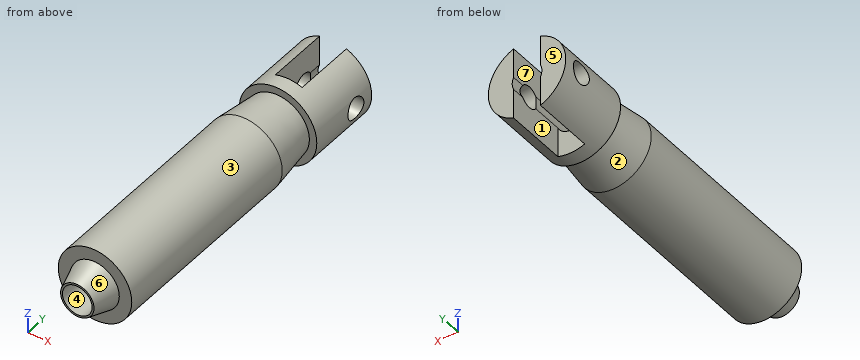
Autodesk Inventor part; units mm, degrees
ref_plane "YZ Plane" through (0, 0, 0) normal (1, 0, 0) x (0, 1, 0)
ref_plane "XZ Plane" through (0, 0, 0) normal (0, 1, 0) x (-1, 0, 0)
ref_plane "XY Plane" through (0, 0, 0) normal (0, 0, 1) x (1, 0, 0)
sketch "Sketch1" plane through (0, 0, 0) normal (0, 0, 1) x (1, 0, 0)
  line L0 (2, 45.442) -> (2, -1.498)
  line L1 (2.254, -1.498) -> (3.2702, 1.754)
  line L2 (3.2702, 1.754) -> (4.953, 1.754)
  line L3 (4.953, 1.754) -> (4.953, 29.3765)
  line L4 (4.953, 29.3765) -> (4.2142, 35.3709)
  line L5 (4.2142, 35.3709) -> (5.2137, 35.3709)
  line L6 (5.2137, 35.3709) -> (5.2137, 45.442)
  line L7 (5.2137, 45.442) -> (2, 45.442)
  line L8 (0, 63.454) -> (0, -29.2362) construction
  line L9 (2.7221, 0) -> (1.4605, -4.0372) construction
  line L10 (1.4605, -4.0372) -> (0, -4.0372) construction
  line L11 (2.254, -1.498) -> (2, -1.498)
  point P0 (0, 0)
  dimension "d0" = 2
  dimension "d1" = 4.953
  dimension "d2" = 3.2702
  dimension "d3" = 43.688
  dimension "d4" = 10.0711
  dimension "d5" = 5.9944
  dimension "d16" = 1.4605
  dimension "d17" = 5.7912
  dimension "d18" = 0.254
revolve "Revolution1" add sketch "Sketch1" angle 360 about axis through (0, 63.454, 0) along (0, -1, 0)
sketch "Sketch2" plane through (0, 45.442, 0) normal (0, 1, 0) x (1, 0, 0)
  line L0 (-1.8097, 6.35) -> (1.8097, 6.35)
  line L1 (1.8097, 6.35) -> (1.8097, -6.35)
  line L2 (1.8097, -6.35) -> (-1.8097, -6.35)
  line L3 (-1.8097, -6.35) -> (-1.8097, 6.35)
  point P0 (0, 0)
  point P1 (0, -6.35)
  point P2 (1.8097, 0)
  dimension "d8" = 3.6195
  dimension "d9" = 12.7
extrude "Extrusion1" cut sketch "Sketch2" against normal blind 8.128
sketch "Sketch3" plane through (1.8097, 45.442, 0.8514) normal (-1, 0, 0) x (0, 0, 1)
  circle A0 centre (-0.8514, -2.8829) radius 1.4605
  line L0 (0, 0) -> (4.0382, 0)
  point P0 (-0.8514, -45.442)
  dimension "d12" = 2.921
  dimension "d13" = 2.8829
extrude "Extrusion2" cut sketch "Sketch3" along normal through all both and the other way through all
properties part number "SolenoidShaft"
For this review, take the finished solid that the model builds, in its own axes (mm). Face numbers are marked on the shaded views. A direction names the side the tool comes from. Round coordinates to 2 decimals unless told otherwise and drop trailing zeros. Order: outer loops, then holes, each group sorted by start corner. A loop starts at its lowest first (then second) coordinate and runs counter-clockwise, first axis right, second up. Notation, with made-up numbers: (9.5, 68) -> (55.5, 68) arc R13 cw to (55.5, 93) -> close; hole circle Ø3 at (42.5, 75). An arc over 180 degrees is marked (long way). Use a Markdown table: item, result.
Item 1: Take a section at D-D (y = 30). State the section outline as (x, z) points, plus the area to 3 significant figures.
Resolved:
| item | result |
|---|---|
| outline | circle Ø9.75 at (0, 0); hole circle Ø4 at (0, 0) |
| area | 62.1 mm² |
Item 2: Take a section at A-A (x = 0). State the section outline as (y, z) points, plus the area to 3 significant figures.
Resolved:
| item | result |
|---|---|
| outline | (-1.5, -2.25) -> (1.75, -3.27) -> (1.75, -4.95) -> (29.38, -4.95) -> (35.37, -4.21) -> (35.37, -5.21) -> (37.31, -5.21) -> (37.31, -2) -> (-1.5, -2) -> close; (-1.5, 2) -> (37.31, 2) -> (37.31, 5.21) -> (35.37, 5.21) -> (35.37, 4.21) -> (29.38, 4.95) -> (1.75, 4.95) -> (1.75, 3.27) -> (-1.5, 2.25) -> close |
| area | 212 mm² |
Item 3: Machinability: for the marked faces 1, 2, 3 and 4, which of the approach directions +Z, -Z, +X, -X, +Y, -Y give a long, thin tool a straight path to every point of the face, cutting with its end or side? Answer none if there is none.
Resolved:
| item | result |
|---|---|
| face 1 | +Z, -Z, +Y |
| face 2 | none |
| face 3 | -Y |
| face 4 | +Y, -Y |
Item 4: Take a section at C-C (y = 20.5). State the section outline as (x, z) points, plus the area to 3 significant figures.
Resolved:
| item | result |
|---|---|
| outline | circle Ø9.91 at (0, 0); hole circle Ø4 at (0, 0) |
| area | 64.5 mm² |
Item 5: Take a section at B-B (z = 0). State the section outline as (x, y) points.
Resolved:
| item | result |
|---|---|
| outline | (-5.21, 35.37) -> (-4.21, 35.37) -> (-4.95, 29.38) -> (-4.95, 1.75) -> (-3.27, 1.75) -> (-2.25, -1.5) -> (-2, -1.5) -> (-2, 41.1) -> (-5.21, 41.1) -> close; (-5.21, 44.02) -> (-2, 44.02) -> (-2, 45.44) -> (-5.21, 45.44) -> close; (2, -1.5) -> (2.25, -1.5) -> (3.27, 1.75) -> (4.95, 1.75) -> (4.95, 29.38) -> (4.21, 35.37) -> (5.21, 35.37) -> (5.21, 41.1) -> (2, 41.1) -> close; (2, 44.02) -> (5.21, 44.02) -> (5.21, 45.44) -> (2, 45.44) -> close |
Item 6: For line 1 along Z through (x, y) = (0, 27.5); line 2 along Y through (x, z) = (-2.25, 2.5); line 3 along Y through (x, z) = (4.75, 1.5), list the stretches that pass through material, from the lowest coordinate up. Write a range as [from, to].
Resolved:
| item | result |
|---|---|
| line 1 | z = [-4.95, -2], [2, 4.95] |
| line 2 | y = [1.75, 45.44] |
| line 3 | y = [35.37, 45.44] |
Item 7: Draft analysis for pull direction X (two halves, no side actions). For the marked faces 5, 6 and 7, state which applies: +X half, -X half, draft (parallel to the pull), parting line (faces both ways), or undercut.
Resolved:
| item | result |
|---|---|
| face 5 | draft |
| face 6 | parting line |
| face 7 | undercut |
Item 8: For pin 1 (1 mm diameter, centred on x = 3.5, y = 8, fed in from -Z); pin 2 (3 mm diameter, centred on x = 0, z = 0, fed in from +Y); pin 3 (2 mm diameter, centred on y = 8, z = -4, fed in from -X); pin 4 (2 mm diameter, centred on y = 42, z = -2, fed in from -X), all flat-tipped, find the tip position at first contact; note any pin that passes through.
Resolved:
| item | result |
|---|---|
| pin 1 | stops at z = -3.94 |
| pin 2 | passes through |
| pin 3 | stops at x = -3.94 |
| pin 4 | stops at x = -5.1 |
